Autodesk Inventor part; units mm, degrees
ref_plane "YZ Plane" through (0, 0, 0) normal (1, 0, 0) x (0, 1, 0)
ref_plane "XZ Plane" through (0, 0, 0) normal (0, 1, 0) x (-1, 0, 0)
ref_plane "XY Plane" through (0, 0, 0) normal (0, 0, 1) x (1, 0, 0)
sketch "Sketch1" plane through (0, 0, 0) normal (0, 1, 0) x (-1, 0, 0)
  line L0 (-15, 10) -> (15, 10)
  line L1 (15, 10) -> (15, -10)
  line L2 (15, -10) -> (-15, -10)
  line L3 (-15, -10) -> (-15, 10)
  line L4 (-15, 10) -> (15, -10) construction
  line L5 (15, 10) -> (-15, -10) construction
  circle A0 centre (10, -5) radius 1.8986
  circle A1 centre (-10, -5) radius 1.8986
  line L6 (10, -3.1013) -> (-10, -3.1013)
  line L7 (10, -6.8986) -> (-10, -6.8986)
  point P0 (0, 0)
  point P1 (0, 0)
  point P2 (10, 0)
  point P3 (0, 0)
  dimension "d0" = 30
  dimension "d1" = 20
  dimension "d8" = 5
  dimension "d61" = 3.7973
  dimension "d62" = 3.7973
  dimension "d63" = 5
  dimension "d64" = 5
  dimension "d67" = 5
extrude "Extrusion1" add sketch "Sketch1" along normal mid plane 7
sketch "Sketch5" plane through (0, 3.5, 0) normal (0, -1, 0) x (1, 0, 0)
  arc A0 (10.771, 2.3227) -> (11.0102, 2.1552) centre (11.0102, 2.4098) ccw
  line L0 (11.0102, 2.1552) -> (11.5022, 2.1552)
  arc A1 (11.5022, 2.1552) -> (11.7414, 2.3227) centre (11.5022, 2.4098) ccw
  line L1 (11.7414, 2.3227) -> (12.7159, 5)
  line L2 (13.7863, 5) -> (12.7159, 5)
  line L3 (13.7863, 5) -> (14.7608, 2.3227)
  arc A2 (14.7608, 2.3227) -> (15, 2.1552) centre (15, 2.4098) ccw
  line L4 (11.5022, 2.4098) -> (15, 2.4098) construction
  line L5 (15, 10) -> (-15, 10) construction
  line L6 (15, -10) -> (15, 10) construction
  line L7 (10.771, 2.3227) -> (10.771, 10)
  line L8 (10.771, 10) -> (15, 10)
  line L9 (15, 10) -> (15, 2.1552)
  dimension "d49" = 0.2546
  dimension "d50" = 0.2546
  dimension "d51" = 0.4921
  dimension "d52" = 1.0704
  dimension "d53" = 2.8448
  dimension "d54" = 3.0194
  dimension "d55" = 0.2546
  dimension "d66" = 5
extrude "Extrusion4" cut sketch "Sketch5" along normal blind 3.5
pattern_linear "Rectangular Pattern1" count 10 spacing 3.99 along (-1, 0, 0) of "Extrusion4"
fillet "Fillet1" radius 2 4 edges at (-15, -1.75, 10) (15, -1.75, 10) (-15, 0, -10) (15, 0, -10)
equation "\"d62\" = d61"
equation "\"d67\" = d64"
equation "\"d55\" = d50"
properties part number "RackTest"
The model under review builds one solid part; all positions refer to its coordinate system, in mm. A direction names the side the tool comes from. Round coordinates to 2 decimals unless told otherwise and drop trailing zeros. Order: outer loops, then holes, each group sorted by start corner. A loop starts at its lowest first (then second) coordinate and runs counter-clockwise, first axis right, second up. Notation, with made-up numbers: (-29.75, 10.5) - (16.25, 10.5) arc R5 cw to (16.25, 19.5) - close; hole circle Ø1 at (-35, 18). An arc over 180 degrees is marked (long way). Use one line per item in the form item = value.
Q1. Add section A-A on z = -5. Give the boundary of the cut face in (x, y), then the cut area to 3 significant figures.
Response values:
outline = (-15, -3.5) - (-11.9, -3.5) - (-11.9, 3.5) - (-15, 3.5) - close; (11.9, -3.5) - (15, -3.5) - (15, 3.5) - (11.9, 3.5) - close
area = 43.4 mm^2
Q2. Add section D-D on z = 7.5. Give the boundary of the cut face in (x, y), then the cut area to 3 significant figures.
Response values:
outline = (-15, -3.5) - (15, -3.5) - (15, 0) - (-15, 0) - close
area = 105 mm^2
Q3. Add section C-C on y = -2.25. Give the boundary of the cut face in (x, z).
Response values:
outline = (-15, -8) arc R2 ccw to (-13, -10) - (13, -10) arc R2 ccw to (15, -8) - (15, 8) arc R2 ccw to (13, 10) - (-13, 10) arc R2 ccw to (-15, 8) - close; hole (-10, -6.9) - (10, -6.9) arc R1.9 ccw to (10, -3.1) - (-10, -3.1) arc R1.9 ccw to start
Q4. Clearance check with flat-ended pins moving along their axes: P1, Ø0.9, axis at x = -10.5, y = 2, coming from the +Z side; P2, Ø4, axis at x = -5.5, z = 7.5, coming from the +Y side. State where each tip first meets the part, or that it passes through.
Response values:
P1 = 5
P2 = 0
Q5. Tool access review of faces 1 (the cylindrical face through (14.43, 0.05, -9.4)), 2 (the cylindrical face through (14.4, -1.73, 9.43)), 3 (the flat face through (-11, 2, 5)), 4 (the flat face through (6.287, 1.774, 3.68)), 5 (the cylindrical face through (-11.9, 0, -5)): name each direction out of +Z, -Z, +X, -X, +Y, -Y from which nothing blocks a thin tool from reaching the whole face with its end or side.
Response values:
face_1 = -Z, +X, +Y, -Y
face_2 = +Z, +X, +Y, -Y
face_3 = +Z, +X, -X, +Y
face_4 = +Z, +Y
face_5 = +Y, -Y
Q6. Mouldability with a two-part tool opening along X and no side actions: class faces 6 (the cylindrical face through (-14.4, -1.77, 9.43)), 7 (the flat face through (14.267, 1.774, 3.68)), 8 (the flat face through (-3.74, 1.77, 3.64)) as pulls with the +X half, pulls with the -X half, needs draft (parallel to the pull), parting line crosses it, or undercut.
Response values:
face_6 = pulls with the -X half
face_7 = pulls with the +X half
face_8 = undercut
Q7. Add section B-B on x = -1.5. Give the boundary of the cut face in (y, z).
Response values:
outline = (-3.5, -10) - (3.5, -10) - (3.5, -6.9) - (-3.5, -6.9) - close; (-3.5, -3.1) - (3.5, -3.1) - (3.5, 3.15) - (0, 3.15) - (0, 10) - (-3.5, 10) - close
Q8. To check wall thickness, follow line 1 (Z direction, x = 5.5, y = -2.5); line 2 (Z direction, x = 9.5, y = 1); line 3 (Y direction, x = 6, z = 6.5). State the ranges of each line that lie inside material, in increasing order.
Response values:
line_1 = -10 to -6.9, -3.1 to 10
line_2 = -10 to -6.9, -3.1 to 5
line_3 = -3.5 to 0
